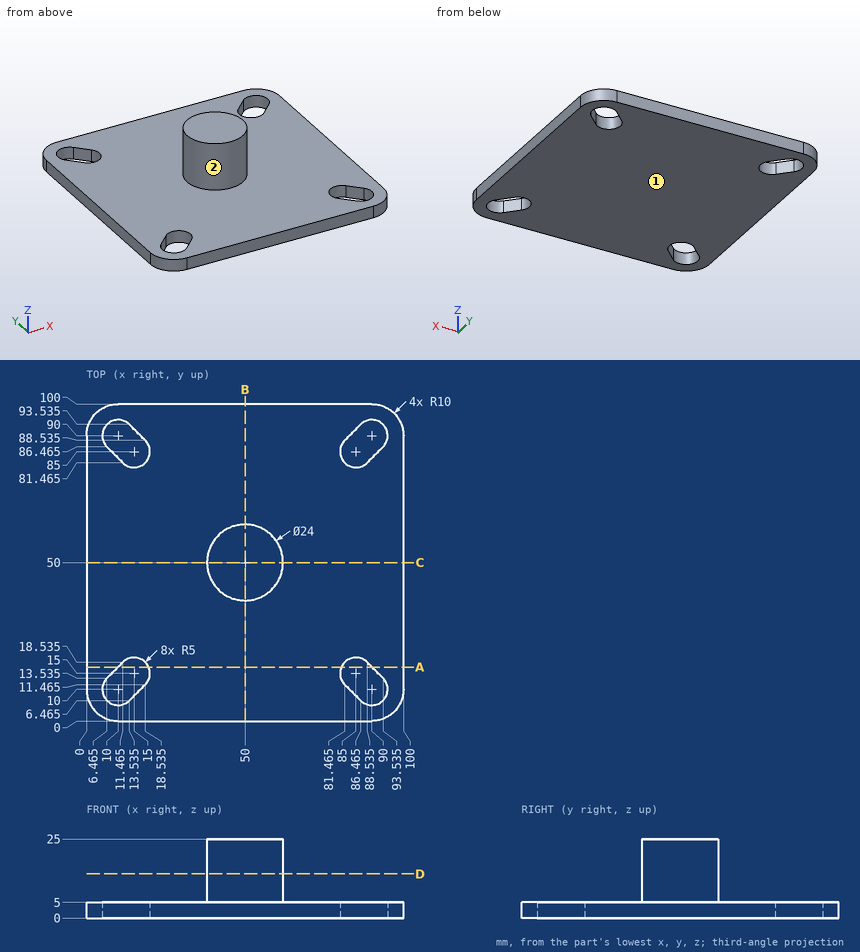
Design review of the part shown in the three views and the two pictorial views. Dimensions are in mm from the part's minimum x, y and z. A direction names the side the tool comes from. Round coordinates to 2 decimals unless told otherwise and drop trailing zeros. Loops run counter-clockwise (first coordinate to the right, second up) from the corner with the lowest first, then second, coordinate; pieces in that order, holes last. Notation, with made-up numbers: M 23,32 L 41,32 A13 cw 41,47 Z; hole C -34.5,56 d9. An arc over 180 degrees is marked long. Answer as a JSON object with one key per item and string values.
Item 1: We need section B-B on x = 50. Give the boundary of the cut face in (y, z), and give its area (3 significant figures).
Answer sheet:
{"outline": "M 0,0 L 100,0 L 100,5 L 62,5 L 62,25 L 38,25 L 38,5 L 0,5 Z", "area": "980 mm^2"}
Item 2: Machinability: for the marked faces 1 and 2, which of the approach directions +Z, -Z, +X, -X, +Y, -Y give a long, thin tool a straight path to every point of the face, cutting with its end or side? Answer none if there is none.
Answer sheet:
{"face 1": "-Z, +X, -X, +Y, -Y", "face 2": "+Z"}
Item 3: We need section D-D on z = 14. Give the boundary of the cut face in (x, y), and give its area (3 significant figures).
Answer sheet:
{"outline": "C 50,50 d24", "area": "452 mm^2"}
Item 4: Wall thickness on L1, parallel to Z at x = 24.5, y = 5.5; L2, parallel to X at y = 61, z = 12.5 (1 decimal); L3, parallel to X at y = 57.5, z = 16 (1 decimal): over which ranges is each line inside the solid? List them lowest first. Write a range as from..to.
Answer sheet:
{"L1": "z = 0..5", "L2": "x = 45.2..54.8", "L3": "x = 40.6..59.4"}
Item 5: Clearance check with flat-ended pins moving along their axes: P1, Ø2, axis at x = 77.5, y = 63, coming from the +Z side; P2, Ø1, axis at y = 61, z = 16, coming from the +X side. State where each tip first meets the part, or that it passes through.
Answer sheet:
{"P1": "stops at z = 5", "P2": "stops at x = 55.81"}
Item 6: We need section A-A on y = 17. Give the boundary of the cut face in (x, z).
Answer sheet:
{"outline": "M 0,0 L 9.93,0 L 9.93,5 L 0,5 Z; M 19.58,0 L 80.42,0 L 80.42,5 L 19.58,5 Z; M 90.07,0 L 100,0 L 100,5 L 90.07,5 Z"}
